```python
from build123d import *

# Parameters (mm, degrees)
BOSS_EXTRUDE1_DEPTH = 3


with BuildPart() as part:
    # Sketch1 → Boss-Extrude1 (new body)
    with BuildSketch(Plane.XY.offset(3)):
        Polygon((22.3672, -1.40536), (22.4409, -0.939999), (22.4852, -0.470929), (22.5, 0), (22.4852, 0.470929), (22.4409, 0.939999), (22.3672, 1.40536), (22.2644, 1.86517), (22.1329, 2.31763), (21.9733, 2.76093), (21.7862, 3.19334), (6.7862, 33.1933), (6.5723, 33.6132), (6.33246, 34.0187), (6.06763, 34.4084), (5.77885, 34.7807), (5.46726, 35.1341), (5.1341, 35.4673), (4.78068, 35.7788), (4.40839, 36.0676), (4.0187, 36.3325), (3.61315, 36.5723), (3.19334, 36.7862), (2.76093, 36.9733), (2.31763, 37.1329), (1.86517, 37.2644), (1.40536, 37.3672), (0.939999, 37.4409), (0.470929, 37.4852), (0, 37.5), (-0.470929, 37.4852), (-0.939999, 37.4409), (-1.40536, 37.3672), (-1.86517, 37.2644), (-2.31763, 37.1329), (-2.76093, 36.9733), (-3.19334, 36.7862), (-3.61315, 36.5723), (-4.0187, 36.3325), (-4.40839, 36.0676), (-4.78068, 35.7788), (-5.1341, 35.4673), (-5.46726, 35.1341), (-5.77885, 34.7807), (-6.06763, 34.4084), (-6.33246, 34.0187), (-6.5723, 33.6132), (-6.7862, 33.1933), (-21.7862, 3.19334), (-21.9733, 2.76093), (-22.1329, 2.31763), (-22.2644, 1.86517), (-22.3672, 1.40536), (-22.4409, 0.939999), (-22.4852, 0.470929), (-22.5, 0), (-22.4852, -0.470929), (-22.4409, -0.939999), (-22.3672, -1.40536), (-22.2644, -1.86517), (-22.1329, -2.31763), (-21.9733, -2.76093), (-21.7862, -3.19334), (-21.5723, -3.61315), (-21.3325, -4.0187), (-21.0676, -4.40839), (-20.7788, -4.78068), (-20.4673, -5.1341), (-20.1341, -5.46726), (-19.7807, -5.77885), (-19.4084, -6.06763), (-19.0187, -6.33246), (-18.6132, -6.5723), (-18.1933, -6.7862), (-17.7609, -6.97332), (-17.3176, -7.13292), (-16.8652, -7.26437), (-16.4054, -7.36715), (-15.94, -7.44086), (-15.4709, -7.4852), (-15, -7.5), (15, -7.5), (15.4709, -7.4852), (15.94, -7.44086), (16.4054, -7.36715), (16.8652, -7.26437), (17.3176, -7.13292), (17.7609, -6.97332), (18.1933, -6.7862), (18.6132, -6.5723), (19.0187, -6.33246), (19.4084, -6.06763), (19.7807, -5.77885), (20.1341, -5.46726), (20.4673, -5.1341), (20.7788, -4.78068), (21.0676, -4.40839), (21.3325, -4.0187), (21.5723, -3.61315), (21.7862, -3.19334), (21.9733, -2.76093), (22.1329, -2.31763), (22.2644, -1.86517), align=None)
        Polygon((0.866025, 1.5), (1.73205, 0), (0.866025, -1.5), (-0.866025, -1.5), (-1.73205, 0), (-0.866025, 1.5), align=None, mode=Mode.SUBTRACT)
        Polygon((-0.866025, 31.5), (0.866025, 31.5), (1.73205, 30), (0.866025, 28.5), (-0.866025, 28.5), (-1.73205, 30), align=None, mode=Mode.SUBTRACT)
        Polygon((15.866, 1.5), (16.7321, 0), (15.866, -1.5), (14.134, -1.5), (13.2679, 0), (14.134, 1.5), align=None, mode=Mode.SUBTRACT)
        Polygon((0.866025, 16.5), (1.73205, 15), (0.866025, 13.5), (-0.866025, 13.5), (-1.73205, 15), (-0.866025, 16.5), align=None, mode=Mode.SUBTRACT)
        Polygon((-14.134, 1.5), (-13.2679, 0), (-14.134, -1.5), (-15.866, -1.5), (-16.7321, 0), (-15.866, 1.5), align=None, mode=Mode.SUBTRACT)
    extrude(amount=-BOSS_EXTRUDE1_DEPTH)


solid = part.part
```
Can you work these out from the model? Positions are in its coordinate system, mm. Give positions to 0.01 mm unless a question says otherwise; leave off trailing zeros. Write each loop counter-clockwise with the first axis right and the second up, starting at its lowest first coordinate (ties: lowest second). Pieces come first, ordered by that corner, then holes. Notation, with made-up numbers: (63.5, -37.5) - (113.5, -37.5) arc R30 ccw to (113.5, -7.5) - close; hole circle Ø8 at (58.25, 53.25). An arc over 180 degrees is marked (long way). Write item = value, one per line. Start each with the question number.
1. Thinking about a two-plate mould opening in Y: for faces 1 (the face through (-15, -1.5, 2)), 2 (the face through (-14.181, 18.403, 1.521)), which applies, released by +Y, released by -Y, zero draft, split by the parting line, or undercut?
2. Imagine slicing it at A-A (z = 0.95). Count the separate pieces of the cut face and the enclosed holes in it, and give its area (3 significant figures).
3. Please list where these lines run through material, in increasing order: line 1 (Y direction, x = 14.5, z = 2.7); line 2 (X direction, y = 15, z = 1.1); line 3 (X direction, y = 1, z = 1).
4. Imagine slicing it at C-C (x = -11.5). Please give me the cut outline in (y, z), and give its area (3 significant figures).
5. For pin 1 (1.4 mm diameter, centred on x = -15, z = 2, fed in from +Y); pin 2 (0.9 mm diameter, centred on x = 15, z = 2, fed in from +Y); pin 3 (3 mm diameter, centred on x = 10.5, y = 32, fed in from -Z), each with a flat end and sliding along its axis, tell me the tip position at first contact or that it passes through.
6. Imagine slicing it at B-B (y = 11.5). Please give me the cut outline in (x, z), and give its area (3 significant figures).
Worked answers:
q1.face_1 = undercut
q1.face_2 = released by +Y
q2.separate_pieces = 1
q2.enclosed_holes = 5
q2.area = 1,320 mm2
q3.line_1 = -7.5 to -1.5, 1.5 to 17.77
q3.line_2 = -15.88 to -1.73, 1.73 to 15.88
q3.line_3 = -22.43 to -16.15, -13.85 to -1.15, 1.15 to 13.85, 16.15 to 22.43
q4.outline = (-7.5, 0) - (23.77, 0) - (23.77, 3) - (-7.5, 3) - close
q4.area = 93.8 mm2
q5.pin_1 = 18.17
q5.pin_2 = 17.67
q5.pin_3 = through
q6.outline = (-17.63, 0) - (17.63, 0) - (17.63, 3) - (-17.63, 3) - close
q6.area = 106 mm2
